Build history of the part. All positions in model axes, mm. Face numbers are marked on the shaded views. A direction names the side the tool comes from. Give positions to 0.01 mm unless a question says otherwise; leave off trailing zeros. Write each loop counter-clockwise with the first axis right and the second up, starting at its lowest first coordinate (ties: lowest second). Pieces come first, ordered by that corner, then holes. Notation, with made-up numbers: (6.25, 26) -> (65.25, 26) arc R31 cw to (65.25, 51) -> close; hole circle Ø11 at (54, -10). An arc over 180 degrees is marked (long way). One line per question, with ' | ' between items. Start each with the question number.
(1) Pull direction X, two halves, no side cores. Call the marked faces 1, 2 and 3: released by +X, released by -X, zero draft, split by the parting line, or undercut.
(2) Tool access for the marked faces 4, 5, 6 and 7: list every direction of +Z, -Z, +X, -X, +Y, -Y with a clear straight run to the whole face (end or side of a thin tool).
(3) Band-saw the part on B-B, the plane y = -6. Give the cut face in (x, z), and give its area (3 significant figures).
(4) Band-saw the part on D-D, the plane y = 12. Give the cut face in (x, z).
(5) Pin check, flat tips, straight feed: P1, Ø1, axis at x = 10, y = -10, coming from the +Z side; P2, Ø5, axis at y = 9.5, z = 2, coming from the +X side; P3, Ø2, axis at y = -1, z = 6.5, coming from the -X side. Stop position of each tip, or through.
(6) Drill centre lines: probe 1 along Y at (x, z) = (0, 0.8); probe 2 along Y at (x, z) = (0, 3.95); probe 3 along Z at (x, y) = (14, 1). Where is each one in solid material? Low to high. Write a range as from..to.
(7) Band-saw the part on C-C, the plane z = 8. Give the cut face in (x, y), and give its area (3 significant figures).
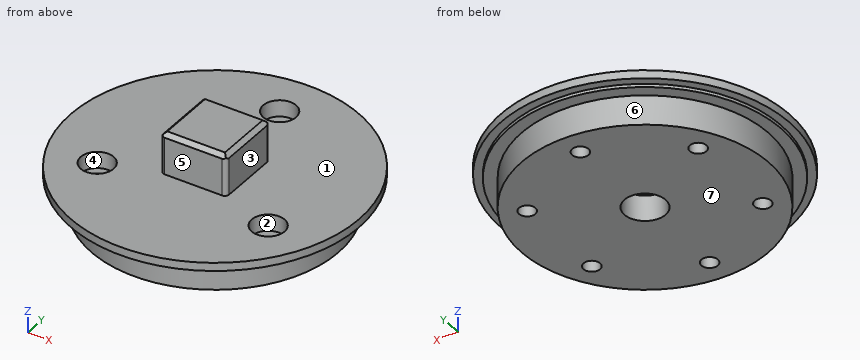
from build123d import *

# Parameters (mm, degrees)
SKETCH_1_R               = 10
EXTRUDE_1_DEPTH          = 4
SKETCH_2_R               = 11.5
EXTRUDE_2_DEPTH          = 1
SKETCH_3_R               = 10.6
EXTRUDE_3_DEPTH          = 0.4
SKETCH_9_R               = 5
CUT_EXTRUDE_5_DEPTH      = 3
SKETCH_10_R              = 12.5
SKETCH_10_R_2            = 11.5
EXTRUDE_4_DEPTH          = 1
SKETCH_11_R              = 5
SKETCH_11_R_2            = 4
EXTRUDE_5_DEPTH          = 3
SKETCH_12_R              = 4
SKETCH_12_R_2            = 2
CUT_EXTRUDE_6_DEPTH      = 1.1
SKETCH_15_R              = 17.5
EXTRUDE_7_DEPTH          = 1
SKETCH_16_R              = 15
SKETCH_16_R_2            = 4
EXTRUDE_9_DEPTH          = 4
SKETCH_17_R              = 1
CUT_EXTRUDE_8_DEPTH      = 2.6
SKETCH_18_R              = 15.5
SKETCH_18_R_2            = 15
EXTRUDE_10_DEPTH         = 0.4
SKETCH_19_R              = 1
CUT_EXTRUDE_9_DEPTH      = 3.6
CUT_EXTRUDE_9_DEPTH_BACK = 3.4
SKETCH_20_R              = 2
CUT_EXTRUDE_10_DEPTH     = 2
SKETCH_21_R              = 16.5
SKETCH_21_R_2            = 15.5
EXTRUDE_11_DEPTH         = 0.4
SKETCH_27_R              = 4
EXTRUDE_12_DEPTH         = 4
SKETCH_38_R              = 1
EXTRUDE_16_DEPTH         = 0.5
SKETCH_40_W              = 8
SKETCH_40_H              = 8
EXTRUDE_18_DEPTH         = 5
CHAMFER_1_SIZE           = 0.5
FILLET_1_R               = 0.5
SKETCH_41_R              = 2.5
CUT_EXTRUDE_11_DEPTH     = 3.1


with BuildPart() as part:
    # 草图1 → 凸台-拉伸1 (new body)
    with BuildSketch(Plane.XY):
        Circle(SKETCH_1_R)
    extrude(amount=EXTRUDE_1_DEPTH)

    # 草图2 → 凸台-拉伸2 (add)
    with BuildSketch(Plane.XY.offset(4)):
        Circle(SKETCH_2_R)
    extrude(amount=EXTRUDE_2_DEPTH)

    # 草图3 → 凸台-拉伸3 (add)
    with BuildSketch(Plane(origin=(0, 0, 4), x_dir=(-1, 0, 0), z_dir=(0, 0, -1))):
        Circle(SKETCH_3_R)
    extrude(amount=EXTRUDE_3_DEPTH)

    # 草图9 → 切除-拉伸5 (cut)
    with BuildSketch(Plane(origin=(0, 0, 0), x_dir=(-1, 0, 0), z_dir=(0, 0, -1))):
        Circle(SKETCH_9_R)
    extrude(amount=-CUT_EXTRUDE_5_DEPTH, mode=Mode.SUBTRACT)

    # 草图10 → 凸台-拉伸4 (add)
    with BuildSketch(Plane.XY.offset(5)):
        Circle(SKETCH_10_R)
        Circle(SKETCH_10_R_2, mode=Mode.SUBTRACT)
    extrude(amount=-EXTRUDE_4_DEPTH)

    # 草图11 → 凸台-拉伸5 (add)
    with BuildSketch(Plane(origin=(0, 0, 3), x_dir=(-1, 0, 0), z_dir=(0, 0, -1))):
        Circle(SKETCH_11_R)
        Circle(SKETCH_11_R_2, mode=Mode.SUBTRACT)
    extrude(amount=EXTRUDE_5_DEPTH)

    # 草图12 → 切除-拉伸6 (cut)
    with BuildSketch(Plane(origin=(0, 0, 3), x_dir=(-1, 0, 0), z_dir=(0, 0, -1))):
        Circle(SKETCH_12_R)
        Circle(SKETCH_12_R_2, mode=Mode.SUBTRACT)
    extrude(amount=-CUT_EXTRUDE_6_DEPTH, mode=Mode.SUBTRACT)

    # 草图15 → 凸台-拉伸7 (add)
    with BuildSketch(Plane.XY.offset(5)):
        Circle(SKETCH_15_R)
    extrude(amount=-EXTRUDE_7_DEPTH)

    # 草图16 → 凸台-拉伸9 (add)
    with BuildSketch(Plane(origin=(0, 0, 4), x_dir=(-1, 0, 0), z_dir=(0, 0, -1))):
        Circle(SKETCH_16_R)
        Circle(SKETCH_16_R_2, mode=Mode.SUBTRACT)
    extrude(amount=EXTRUDE_9_DEPTH)

    # 草图17 → 切除-拉伸8 (cut)
    with BuildSketch(Plane(origin=(0, 0, 0), x_dir=(-1, 0, 0), z_dir=(0, 0, -1))):
        with Locations((0, 12)):
            Circle(SKETCH_17_R)
        with Locations((10.392304845, 6)):
            Circle(SKETCH_17_R)
        with Locations((10.392304845, -6)):
            Circle(SKETCH_17_R)
        with Locations((0, -12)):
            Circle(SKETCH_17_R)
        with Locations((-10.392304845, -6)):
            Circle(SKETCH_17_R)
        with Locations((-10.392304845, 6)):
            Circle(SKETCH_17_R)
    extrude(amount=-CUT_EXTRUDE_8_DEPTH, mode=Mode.SUBTRACT)

    # 草图18 → 凸台-拉伸10 (add)
    with BuildSketch(Plane(origin=(0, 0, 4), x_dir=(-1, 0, 0), z_dir=(0, 0, -1))):
        Circle(SKETCH_18_R)
        Circle(SKETCH_18_R_2, mode=Mode.SUBTRACT)
    extrude(amount=EXTRUDE_10_DEPTH)

    # 草图19 → 切除-拉伸9 (cut, two sides)
    with BuildSketch(Plane(origin=(0, 0, 2.6), x_dir=(-1, 0, 0), z_dir=(0, 0, -1))) as cut_extrude_9_sk:
        with Locations((0, 12)):
            Circle(SKETCH_19_R)
        with Locations((10.392304845, -6)):
            Circle(SKETCH_19_R)
        with Locations((-10.392304845, -6)):
            Circle(SKETCH_19_R)
    extrude(amount=CUT_EXTRUDE_9_DEPTH, mode=Mode.SUBTRACT)
    extrude(cut_extrude_9_sk.sketch, amount=-CUT_EXTRUDE_9_DEPTH_BACK, mode=Mode.SUBTRACT)

    # 草图20 → 切除-拉伸10 (cut)
    with BuildSketch(Plane.XY.offset(5)):
        with Locations((0, 12)):
            Circle(SKETCH_20_R)
        with Locations((10.392304845, -6)):
            Circle(SKETCH_20_R)
        with Locations((-10.392304845, -6)):
            Circle(SKETCH_20_R)
    extrude(amount=-CUT_EXTRUDE_10_DEPTH, mode=Mode.SUBTRACT)

    # 草图21 → 凸台-拉伸11 (add)
    with BuildSketch(Plane(origin=(0, 0, 3.6), x_dir=(-1, 0, 0), z_dir=(0, 0, -1))):
        Circle(SKETCH_21_R)
        Circle(SKETCH_21_R_2, mode=Mode.SUBTRACT)
    extrude(amount=-EXTRUDE_11_DEPTH)

    # 草图27 → 凸台-拉伸12 (add)
    with BuildSketch(Plane(origin=(0, 0, 0), x_dir=(-1, 0, 0), z_dir=(0, 0, -1))):
        Circle(SKETCH_27_R)
    extrude(amount=-EXTRUDE_12_DEPTH)

    # 草图38 → 凸台-拉伸16 (add)
    with BuildSketch(Plane(origin=(0, 0, 2.6), x_dir=(-1, 0, 0), z_dir=(0, 0, -1))):
        with Locations((10.392304845, 6)):
            Circle(SKETCH_38_R)
        with Locations((0, -12)):
            Circle(SKETCH_38_R)
        with Locations((-10.392304845, 6)):
            Circle(SKETCH_38_R)
    extrude(amount=EXTRUDE_16_DEPTH)

    # 草图40 → 凸台-拉伸18 (add)
    with BuildSketch(Plane.XY.offset(5)):
        Rectangle(SKETCH_40_W, SKETCH_40_H)
    extrude(amount=EXTRUDE_18_DEPTH)

    # 倒角1
    chamfer_1_edges = [part.edges().sort_by_distance(p)[0] for p in [
        (-4, 0, 10),
        (0, -4, 10),
        (4, 0, 10),
        (0, 4, 10),
    ]]
    chamfer(chamfer_1_edges, length=CHAMFER_1_SIZE)

    # 圆角1
    fillet_1_edges = [part.edges().sort_by_distance(p)[0] for p in [
        (-4, 4, 7.25),
        (4, 4, 7.25),
        (4, -4, 7.25),
        (-4, -4, 7.25),
    ]]
    fillet(fillet_1_edges, radius=FILLET_1_R)

    # 草图41 → 切除-拉伸11 (cut)
    with BuildSketch(Plane(origin=(0, 0, 0), x_dir=(-1, 0, 0), z_dir=(0, 0, -1))):
        Circle(SKETCH_41_R)
    extrude(amount=-CUT_EXTRUDE_11_DEPTH, mode=Mode.SUBTRACT)


solid = part.part
Results:
1) face 1: zero draft | face 2: undercut | face 3: released by +X
2) face 4: +Z | face 5: +Z, +X, -X, -Y | face 6: -Z | face 7: -Z, +X, -X, +Y, -Y
3) outline: (-16.44, 4) -> (-15.37, 4) -> (-15.37, 3.6) -> (-13.75, 3.6) -> (-13.75, 0) -> (-11.39, 0) -> (-11.39, 3) -> (-12.39, 3) -> (-12.39, 5) -> (-16.44, 5) -> close; (-9.39, 0) -> (9.39, 0) -> (9.39, 3) -> (8.39, 3) -> (8.39, 5) -> (-8.39, 5) -> (-8.39, 3) -> (-9.39, 3) -> close; (11.39, 0) -> (13.75, 0) -> (13.75, 3.6) -> (15.37, 3.6) -> (15.37, 4) -> (16.44, 4) -> (16.44, 5) -> (12.39, 5) -> (12.39, 3) -> (11.39, 3) -> close | area: 116 mm²
4) outline: (-12.74, 4) -> (-11.32, 4) -> (-11.32, 3.6) -> (-9, 3.6) -> (-9, 0) -> (-1, 0) -> (-1, 3) -> (-2, 3) -> (-2, 5) -> (-12.74, 5) -> close; (1, 0) -> (9, 0) -> (9, 3.6) -> (11.32, 3.6) -> (11.32, 4) -> (12.74, 4) -> (12.74, 5) -> (2, 5) -> (2, 3) -> (1, 3) -> close
5) P1: stops at z = 5 | P2: stops at x = 15.56 | P3: stops at x = -4
6) probe 1: y = -15..-13, -11..-2.5, 2.5..11, 13..15 | probe 2: y = -16.5..10, 14..16.5 | probe 3: z = 0..5
7) outline: (-4, -3.5) arc R0.5 ccw to (-3.5, -4) -> (3.5, -4) arc R0.5 ccw to (4, -3.5) -> (4, 3.5) arc R0.5 ccw to (3.5, 4) -> (-3.5, 4) arc R0.5 ccw to (-4, 3.5) -> close | area: 63.8 mm²
